```python
from build123d import *

# Parameters (mm, degrees)
CROQUIS1_W              = 440
CROQUIS1_H              = 330
SALIENTE_EXTRUIR1_DEPTH = 20
CROQUIS3_R              = 4
SALIENTE_EXTRUIR2_DEPTH = 100
CROQUIS5_R              = 2.5
CORTAR_EXTRUIR2_DEPTH   = 100
CROQUIS3_3_R            = 2.5
SALIENTE_EXTRUIR3_DEPTH = 225
CROQUIS3_4_R            = 2.5
SALIENTE_EXTRUIR4_DEPTH = 255
CROQUIS3_5_R            = 2.5
SALIENTE_EXTRUIR5_DEPTH = 255
CROQUIS3_6_R            = 2.5
SALIENTE_EXTRUIR6_DEPTH = 285
CROQUIS3_7_R            = 2.5
SALIENTE_EXTRUIR7_DEPTH = 320


with BuildPart() as part:
    # Croquis1 → Saliente-Extruir1 (new body)
    with BuildSketch(Plane.XY):
        with Locations((220, 165)):
            Rectangle(CROQUIS1_W, CROQUIS1_H)
    extrude(amount=SALIENTE_EXTRUIR1_DEPTH)

    # Croquis3 → Saliente-Extruir2 (add)
    with BuildSketch(Plane.XY.offset(20)):
        with Locations((70, 180)):
            Circle(CROQUIS3_R)
    extrude(amount=SALIENTE_EXTRUIR2_DEPTH)

    # Croquis5 → Cortar-Extruir2 (cut)
    with BuildSketch(Plane.XY.offset(120)):
        with Locations((70, 180)):
            Circle(CROQUIS5_R)
    extrude(amount=-CORTAR_EXTRUIR2_DEPTH, mode=Mode.SUBTRACT)

    # Croquis3<3> → Saliente-Extruir3 (add)
    with BuildSketch(Plane.XY.offset(20)):
        with Locations((136, 180)):
            Circle(CROQUIS3_3_R)
    extrude(amount=SALIENTE_EXTRUIR3_DEPTH)

    # Croquis3<4> → Saliente-Extruir4 (add)
    with BuildSketch(Plane.XY.offset(20)):
        with Locations((203.2, 180)):
            Circle(CROQUIS3_4_R)
    extrude(amount=SALIENTE_EXTRUIR4_DEPTH)

    # Croquis3<5> → Saliente-Extruir5 (add)
    with BuildSketch(Plane.XY.offset(20)):
        with Locations((203.2, 180)):
            Circle(CROQUIS3_5_R)
    extrude(amount=SALIENTE_EXTRUIR5_DEPTH)

    # Croquis3<6> → Saliente-Extruir6 (add)
    with BuildSketch(Plane.XY.offset(20)):
        with Locations((256.5, 180)):
            Circle(CROQUIS3_6_R)
    extrude(amount=SALIENTE_EXTRUIR6_DEPTH)

    # Croquis3<7> → Saliente-Extruir7 (add)
    with BuildSketch(Plane.XY.offset(20)):
        with Locations((307, 180)):
            Circle(CROQUIS3_7_R)
        with Locations((368, 180)):
            Circle(CROQUIS3_7_R)
    extrude(amount=SALIENTE_EXTRUIR7_DEPTH)


solid = part.part
```
Verification items for the finished model (mm, model axes). Coordinates: 2 decimals unless noted, no trailing zeros. Order: outer loops, then holes, each group sorted by start corner. A loop starts at its lowest first (then second) coordinate and runs counter-clockwise, first axis right, second up. Notation, with made-up numbers: (-7.75, -31.75) - (41.25, -31.75) arc R11 ccw to (41.25, -16.75) - close; hole circle Ø1 at (32, 7). An arc over 180 degrees is marked (long way). Return JSON: item names as keys, results as strings.
(1) Section check A-A, the plane z = 69.5. Record the cut outline in (x, y).
Filled sheet:
{"outline": "circle Ø8 at (70, 180); circle Ø5 at (136, 180); circle Ø5 at (203.2, 180); circle Ø5 at (256.5, 180); circle Ø5 at (307, 180); circle Ø5 at (368, 180); hole circle Ø5 at (70, 180)"}
(2) Thickness scan on line 1 along Y through (x, z) = (70, 41); line 2 along Z through (x, y) = (70, 29); line 3 along Y through (x, z) = (309, 65). Record the ranges inside material, lowest first.
Filled sheet:
{"line 1": "y = 176 to 177.5, 182.5 to 184", "line 2": "z = 0 to 20", "line 3": "y = 178.5 to 181.5"}
(3) Go/stop test with flat-tipped pins: pin 1 (5.5 mm diameter, centred on x = 257, y = 179.5, fed in from +Z); pin 2 (6 mm diameter, centred on x = 213, y = 198.5, fed in from +Z); pin 3 (6.5 mm diameter, centred on x = 69, y = 180.5, fed in from +Z). Record where each tip stops, or that it passes through.
Filled sheet:
{"pin 1": "stops at z = 305", "pin 2": "stops at z = 20", "pin 3": "stops at z = 120"}
(4) Section check D-D, the plane y = 137. Record the cut outline in (x, z), and give its area (3 significant figures).
Filled sheet:
{"outline": "(0, 0) - (440, 0) - (440, 20) - (0, 20) - close", "area": "8,800 mm^2"}
(5) Section check B-B, the plane z = 231. Record the cut outline in (x, y).
Filled sheet:
{"outline": "circle Ø5 at (136, 180); circle Ø5 at (203.2, 180); circle Ø5 at (256.5, 180); circle Ø5 at (307, 180); circle Ø5 at (368, 180)"}
(6) Section check C-C, the plane x = 228.5. Record the cut outline in (y, z).
Filled sheet:
{"outline": "(0, 0) - (330, 0) - (330, 20) - (0, 20) - close"}
